Verification items for the finished model (mm, model axes). Face numbers are marked on the shaded views. A direction names the side the tool comes from. Coordinates: 2 decimals unless noted, no trailing zeros. Write each loop counter-clockwise with the first axis right and the second up, starting at its lowest first coordinate (ties: lowest second). Pieces come first, ordered by that corner, then holes. Notation, with made-up numbers: (-39, 42) - (-25, 42) arc R30 cw to (-25, 79) - close; hole circle Ø2 at (59, -5.75). An arc over 180 degrees is marked (long way). Use one line per item in the form item = value. Start each with the question number.
(1) Sectioned sample at C-C (z = -61). Record the cut outline in (x, y).
(2) Gauge pin test, flat ends, axial feed: pin 1 Ø3.5 at (x, z) = (47.5, -56.68) entering from -Y; pin 2 Ø2 at (x, y) = (2.5, 22) entering from +Z; pin 3 Ø12 at (x, z) = (19.5, -63) entering from +Y; pin 4 Ø7.5 at (y, z) = (4, -23) entering from +X. Record the tip position at first contact, or that the pin passes through.
(3) Sectioned sample at B-B (y = 8.5). Record the cut outline in (x, z).
(4) Material ranges on line 1 (X direction, y = 8, z = -20); line 2 (X direction, y = 9, z = -9.5); line 3 (Y direction, x = 53, z = -22), recorded low to high. Write a range as [from, to].
(5) Tool access check on the marked faces 1, 2 and 3. Record the directions out of +Z, -Z, +X, -X, +Y, -Y that give a thin tool (end or side, any length) a straight path to the whole face; none if there is none.
(6) Mould release check, pull along Y, two halves, no side actions. Record for the marked faces 4, 5, 6 and 7: released by +Y, released by -Y, zero draft, split by the parting line, or undercut.
(7) Sectioned sample at A-A (y = 65.8). Record the cut outline in (x, z).
(8) Sectioned sample at D-D (x = 22). Count the separate pieces of the cut face and the enclosed holes in it, and give its area (3 significant figures).
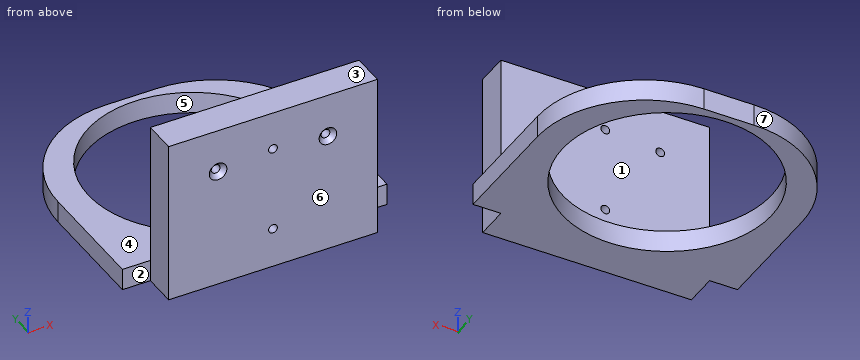
Autodesk Inventor part; units mm, degrees
ref_plane "YZ Plane" through (0, 0, 0) normal (1, 0, 0) x (0, 1, 0)
ref_plane "XZ Plane" through (0, 0, 0) normal (0, 1, 0) x (-1, 0, 0)
ref_plane "XY Plane" through (0, 0, 0) normal (0, 0, 1) x (1, 0, 0)
sketch "Sketch1" plane through (0, 0, 0) normal (0, 1, 0) x (-1, 0, 0)
  line L0 (0, 0) -> (-94.996, 0)
  line L1 (-94.996, 0) -> (-94.996, -75)
  line L2 (-94.996, -75) -> (0, -75)
  line L3 (0, -75) -> (0, 0)
  dimension "d0" = 94.996
  dimension "d1" = 75
extrude "Extrusion1" add sketch "Sketch1" along normal blind 15
sketch "Sketch2" plane through (0, 15, 0) normal (0, 1, 0) x (1, 0, 0)
  line L0 (94.996, 75) -> (0, 75)
  line L1 (0, 75) -> (-12.7, 75)
  line L2 (94.996, 0) -> (94.996, 75)
  line L3 (94.996, 75) -> (107.696, 75)
  line L4 (107.696, 75) -> (107.696, 65.094)
  line L5 (107.696, 65.094) -> (-12.7, 65.094)
  line L6 (-12.7, 65.094) -> (-12.7, 75)
  line L7 (0, 75) -> (94.996, 75)
  point P0 (0, 0)
  dimension "d4" = 12.7
  dimension "d5" = 12.7
  dimension "d6" = 9.906
extrude "Extrusion2" add sketch "Sketch2" along normal blind 101.6
sketch "Sketch4" plane through (0, 0, 0) normal (0, -1, 0) x (1, 0, 0)
  line L0 (0, 0) -> (94.996, 0)
  line L1 (94.996, -75) -> (0, -75)
  circle A0 centre (47.498, -17.5525) radius 2
  circle A1 centre (47.498, -56.6788) radius 2
  dimension "d12" = 4
  dimension "d13" = 4
extrude "Extrusion4" cut sketch "Sketch4" against normal through all
sketch "Sketch5" plane through (-12.7, 15, -65.094) normal (0, 0, 1) x (1, 0, 0)
  line L0 (58.198, 0) -> (62.198, 0)
  line L1 (120.396, 0) -> (120.396, 101.6)
  circle A0 centre (60.198, 50.8) radius 47.5
  point P0 (12.7, -15)
  dimension "d17" = 95
extrude "Extrusion5" cut sketch "Sketch5" against normal through all
sketch "Sketch6" plane through (0, 15, 0) normal (0, 1, 0) x (1, 0, 0)
  line L0 (0, 0) -> (94.996, 0)
  circle A0 centre (72.498, 20) radius 2
  circle A1 centre (22.498, 20) radius 2
  dimension "d23" = 4
extrude "Extrusion6" cut sketch "Sketch6" against normal through all
chamfer "Chamfer1" distance 2 angle 45 2 edges at (70.498, 0, -20) (20.498, 0, -20)
fillet "Fillet1" radius 48.75 2 edges at (-12.7, 116.6, -70.047) (107.696, 116.6, -70.047)
properties part number "Harmonic Drive Mount"
Answers below:
q1.outline = (0, 0) - (95, 0) - (95, 15) - (0, 15) - close
q2.pin_1 = through
q2.pin_2 = -65.09
q2.pin_3 = 115.36
q2.pin_4 = 95
q3.outline = (0, -75) - (95, -75) - (95, 0) - (0, 0) - close; hole circle Ø4 at (22.5, -20); hole circle Ø4 at (47.5, -56.68); hole circle Ø4 at (47.5, -17.55); hole circle Ø4 at (72.5, -20)
q4.line_1 = [0, 20.5], [24.5, 70.5], [74.5, 95]
q4.line_2 = [0, 95]
q4.line_3 = [0, 15]
q5.face_1 = +Z, +X, -X, +Y
q5.face_2 = +Z, -Z, -X, -Y
q5.face_3 = +Z, +X, -X, +Y, -Y
q6.face_4 = zero draft
q6.face_5 = undercut
q6.face_6 = released by -Y
q6.face_7 = released by +Y
q7.outline = (-12.7, -75) - (0, -75) - (0, -65.09) - (-12.7, -65.09) - close; (95, -75) - (107.7, -75) - (107.7, -65.09) - (95, -65.09) - close
q8.separate_pieces = 3
q8.enclosed_holes = 0
q8.area = 1,250 mm2
